Could you check a few things on this model? Use its own coordinates, in mm. Face numbers are marked on the shaded views. A direction names the side the tool comes from. Give positions to 0.01 mm unless a question says otherwise; leave off trailing zeros. Write each loop counter-clockwise with the first axis right and the second up, starting at its lowest first coordinate (ties: lowest second). Pieces come first, ordered by that corner, then holes. Notation, with made-up numbers: (2.5, 84) - (6.5, 84) arc R13 ccw to (6.5, 101) - close; hole circle Ø8 at (34, 37). An arc over 180 degrees is marked (long way). Use one line per item in the form item = value.
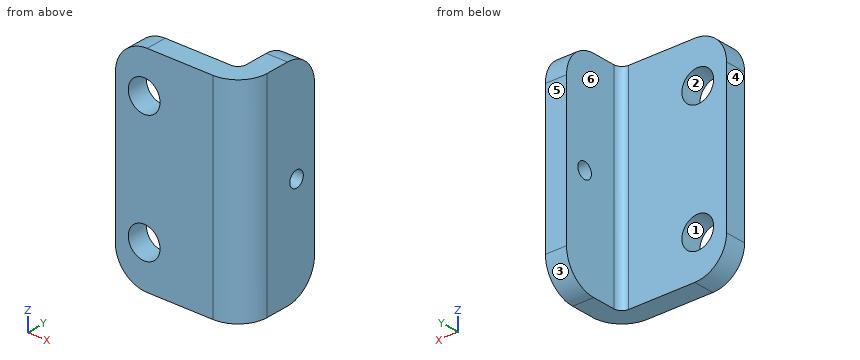
```python
from build123d import *

# Parameters (mm, degrees)
BASE_FLANGE1_DEPTH = 10
FILLET1_R          = 3
SKETCH6_R          = 1.5
CUT_EXTRUDE1_DEPTH = 17.733200531
SKETCH7_R          = 0.75
CUT_EXTRUDE2_DEPTH = 17.248076809


# Sheet-metal steps are written as plain solids
with BuildPart() as part:
    # Sketch1 → Base-Flange1 (new, symmetric)
    with BuildSketch(Plane.XY):
        with BuildLine():
            Line((0, 8), (0, 2.75))
            ThreePointArc((0, 2.75), (-0.805456352, 0.805456352), (-2.75, 0))
            Line((-2.75, 0), (-12, 0))
            Line((-12, 0), (-12, 2))
            Line((-12, 2), (-2.75, 2))
            ThreePointArc((-2.75, 2), (-2.219669914, 2.219669914), (-2, 2.75))
            Line((-2, 2.75), (-2, 8))
            Line((-2, 8), (0, 8))
        make_face()
    extrude(amount=BASE_FLANGE1_DEPTH, both=True)

    # Fillet1
    fillet1_edges = [part.edges().sort_by_distance(p)[0] for p in [
        (-1, 8, 10),
        (-12, 1, 10),
        (-1, 8, -10),
        (-12, 1, -10),
    ]]
    fillet(fillet1_edges, radius=FILLET1_R)

    # Sketch6 → Cut-Extrude1 (cut, through all)
    with BuildSketch(Plane(origin=(0, 2, 0), x_dir=(1, 0, 0), z_dir=(0, 1, 0))):
        with Locations(Location((-9.278968908, 6, 0), (0, 0, 180))):
            Circle(SKETCH6_R)
        with Locations((-9.278968908, -6)):
            Circle(SKETCH6_R)
    extrude(amount=-CUT_EXTRUDE1_DEPTH, mode=Mode.SUBTRACT)

    # Sketch7 → Cut-Extrude2 (cut, through all)
    with BuildSketch(Plane.ZY.offset(2)):
        with Locations((0, 6)):
            Circle(SKETCH7_R)
    extrude(amount=-CUT_EXTRUDE2_DEPTH, mode=Mode.SUBTRACT)


solid = part.part
```
1. For pin 1 (4 mm diameter, centred on x = -10.5, z = -1.5, fed in from -Y); pin 2 (1 mm diameter, centred on x = -7.5, z = -8, fed in from +Y), each with a flat end and sliding along its axis, tell me the tip position at first contact or that it passes through.
Response values:
pin_1 = 0
pin_2 = 2
2. Which directions (+Z, -Z, +X, -X, +Y, -Y) give clear straight access to the entire face, cutting with the end or side of a thin tool? Please do the marked faces 5 and 6.
Response values:
face_5 = +Z, -Z, +X, -X, +Y
face_6 = +Z, -Z, -X, +Y
3. Imagine slicing it at A-A, the plane z = 6. List the corners of the cut face in (x, y) for me.
Response values:
outline = (-12, 0) - (-10.78, 0) - (-10.78, 2) - (-12, 2) - close; (-7.78, 0) - (-2.75, 0) arc R2.75 ccw to (0, 2.75) - (0, 8) - (-2, 8) - (-2, 2.75) arc R0.75 cw to (-2.75, 2) - (-7.78, 2) - close
4. If I drill on line 1 (Y direction, x = -4.75, z = -9); line 2 (X direction, y = 5, z = -7); line 3 (Y direction, x = -1.15, z = 0), over which ranges is the centre line in solid material (lowest first)? Write a range as from..to.
Response values:
line_1 = 0..2
line_2 = -2..0
line_3 = 0.51..5.25, 6.75..8
5. Imagine slicing it at B-B, the plane y = 5.5. List the corners of the cut face in (x, z) for me, and give its area (3 significant figures).
Response values:
outline = (-2, -9.96) - (0, -9.96) - (0, -0.56) - (-2, -0.56) - close; (-2, 0.56) - (0, 0.56) - (0, 9.96) - (-2, 9.96) - close
area = 37.6 mm²
6. Imagine slicing it at D-D, the plane y = 1. List the corners of the cut face in (x, z) for me, and give its area (3 significant figures).
Response values:
outline = (-12, -7) arc R3 ccw to (-9, -10) - (-0.63, -10) - (-0.63, 10) - (-9, 10) arc R3 ccw to (-12, 7) - close; hole circle Ø3 at (-9.28, -6); hole circle Ø3 at (-9.28, 6)
area = 209 mm²
7. If we mould it in two halves opening along Z, with no side actions, what happens to the marked faces 1, 2, 3 and 4? For each: pulls with the +Z half, pulls with the -Z half, needs draft (parallel to the pull), parting line crosses it, or undercut.
Response values:
face_1 = undercut
face_2 = undercut
face_3 = pulls with the -Z half
face_4 = needs draft
8. Imagine slicing it at C-C, the plane x = -10.5. List the corners of the cut face in (y, z) for me, and give its area (3 significant figures).
Response values:
outline = (0, -9.6) - (2, -9.6) - (2, -6.87) - (0, -6.87) - close; (0, -5.13) - (2, -5.13) - (2, 5.13) - (0, 5.13) - close; (0, 6.87) - (2, 6.87) - (2, 9.6) - (0, 9.6) - close
area = 31.4 mm²
